from build123d import *

# Parameters (mm, degrees)
BOSS_EXTRUDE1_DEPTH = 3
SKETCH2_R           = 2.25
BOSS_EXTRUDE2_DEPTH = 82


with BuildPart() as part:
    # Sketch1 → Boss-Extrude1 (new body)
    with BuildSketch(Plane(origin=(0, 0, 0), x_dir=(1, 0, 0), z_dir=(0, 1, 0))):
        Polygon((-4.5, 0), (-2.25, -3.897114317), (2.25, -3.897114317), (4.5, 0), (2.25, 3.897114317), (-2.25, 3.897114317), align=None)
    extrude(amount=BOSS_EXTRUDE1_DEPTH)

    # Sketch2 → Boss-Extrude2 (add)
    with BuildSketch(Plane(origin=(0, 3, 0), x_dir=(1, 0, 0), z_dir=(0, 1, 0))):
        Circle(SKETCH2_R)
    extrude(amount=BOSS_EXTRUDE2_DEPTH)

    # Sketch4 → Cut-Revolve1 (revolve, cut)
    with BuildSketch(Plane(origin=(0, 0, 0), x_dir=(0, 0, -1), z_dir=(1, 0, 0))):
        Polygon((3.897114317, 0), (4.897114317, 1), (4.897114317, 0), align=None)
    revolve(axis=Axis((0, 0, 0), (0, 1, 0)), mode=Mode.SUBTRACT)


solid = part.part
Here's how the part is built. I have some questions about the finished solid (model axes, mm). A direction names the side the tool comes from. Coordinates: 2 decimals unless noted, no trailing zeros. Order: outer loops, then holes, each group sorted by start corner. A loop starts at its lowest first (then second) coordinate and runs counter-clockwise, first axis right, second up. Notation, with made-up numbers: M 71.25,85.25 L 115.25,85.25 A22 cw 115.25,106.25 Z; hole C -37.75,50 d11. An arc over 180 degrees is marked long. Answer as CSV lines item,"result". Start each with the question number.
1. I need wall thicknesses on line 1 (Y direction, x = 2.25, z = -3); line 2 (Z direction, x = 0, y = 61.5); line 3 (X direction, y = 44, z = 0.5). Which ranges of each line are inside material? Lowest first, please. Write a range as [from, to].
2. For pin 1 (3 mm diameter, centred on y = 14, z = 0, fed in from -X); pin 2 (3 mm diameter, centred on y = 55.5, z = 1.5, fed in from +X); pin 3 (4 mm diameter, centred on x = -2.5, y = 59, fed in from +Z), each with a flat end and sliding along its axis, tell me the tip position at first contact or that it passes through.
3. I want a section at A-A, the plane y = 56.5. Write out the boundary of the cut face in (x, z).
4. On a 3-axis mill with a long thin cutter (end or side, diameter ignored), from which of +Z, -Z, +X, -X, +Y, -Y can I reach the whole of each face in a straight line? I mean faces 1 (the flat face through (0, 1, 3.897)), 2 (the cylindrical face through (-0.29, 43.43, -2.23)). Say none if no direction works.
Recorded:
1,line 1,"y = [0, 3]"
1,line 2,"z = [-2.25, 2.25]"
1,line 3,"x = [-2.19, 2.19]"
2,pin 1,"stops at x = -2.25"
2,pin 2,"stops at x = 2.25"
2,pin 3,"stops at z = 2.19"
3,outline,"C 0,0 d4.5"
4,face 1,"+Z, +X, -X, +Y, -Y"
4,face 2,"+Y"
